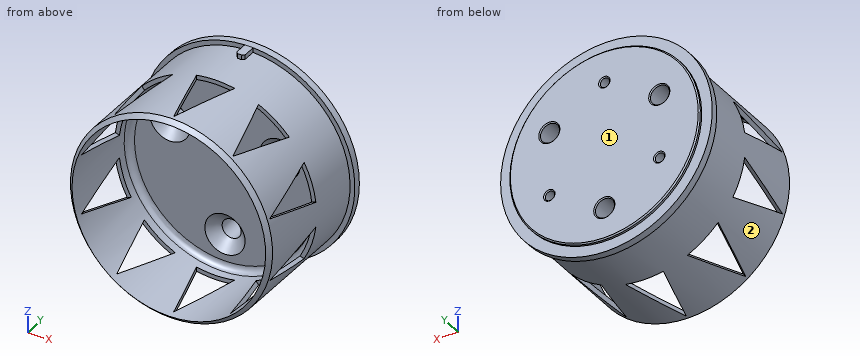
from build123d import *

# Parameters (mm, degrees)
CUT_EXTRUDE_651_DEPTH      = 70.85
PATTERN_CIRCULAR_705_COUNT = 5
SKETCH_7_R                 = 50
EXTRUDE_1_DEPTH            = 5
CUT_EXTRUDE_START          = -1.6
SKETCH_8_R                 = 50
SKETCH_8_R_2               = 45
CUT_EXTRUDE_1_DEPTH        = 1.6
SKETCH_10_R                = 4.5
CUT_EXTRUDE_4_DEPTH        = 97.046863561
SKETCH_10_4_R              = 2.2
CUT_EXTRUDE_5_DEPTH        = 8
CHAMFER_1_SIZE             = 0.5
EXTRUDE_START              = 7
EXTRUDE_2_DEPTH            = 7
CHAMFER_4_SIZE             = 1
CHAMFER_5_SIZE             = 2
CHAMFER_6_SIZE             = 5
CHAMFER_7_SIZE             = 0.6


with BuildPart() as part:
    # Эскиз2 → Revolve 379 (revolve)
    with BuildSketch(Plane.XY, mode=Mode.PRIVATE) as revolve_379_sk:
        with BuildLine():
            Line((0, 0), (-47.75, 0))
            Line((-47.75, 0), (-47.75, -60))
            Line((-47.75, -60), (-45.75, -60))
            Line((-45.75, -60), (-45.75, -21))
            ThreePointArc((-45.75, -21), (-44.871320344, -18.878679656), (-42.75, -18))
            Line((-42.75, -18), (0, -18))
            Line((0, -18), (0, 0))
        make_face()
    revolve(revolve_379_sk.sketch.rotate(Axis((0, 0, 0), (0, 1, 0)), 270), axis=Axis((0, 0, 0), (0, 1, 0)))

    # Эскиз4 → Cut-Extrude 651 (cut, symmetric)
    with BuildSketch(Plane.XY):
        Polygon((-9, -25), (9, -25), (0, -56.5), align=None)
    cut_extrude_651 = extrude(amount=CUT_EXTRUDE_651_DEPTH, both=True, mode=Mode.SUBTRACT)

    # Pattern Circular 705: Cut-Extrude 651 ×5 about axis
    pattern_circular_705_axis = Axis((0, 0, 0), (0, 1, 0))
    for i in range(1, PATTERN_CIRCULAR_705_COUNT):
        add(cut_extrude_651.rotate(pattern_circular_705_axis, i * 360 / PATTERN_CIRCULAR_705_COUNT), mode=Mode.SUBTRACT)

    # Эскиз7 → Бобышка-Вытянуть1 (add)
    with BuildSketch(Plane(origin=(0, 0, 0), x_dir=(1, 0, 0), z_dir=(0, 1, 0))):
        with Locations(Location((0, 0, 0), (0, 0, 270))):
            Circle(SKETCH_7_R)
    extrude(amount=EXTRUDE_1_DEPTH)

    # Эскиз8 → Вырез-Вытянуть1 (cut)
    with BuildSketch(Plane(origin=(0, 5, 0), x_dir=(1, 0, 0), z_dir=(0, 1, 0)).offset(CUT_EXTRUDE_START)):
        with Locations(Location((0, 0, 0), (0, 0, 270))):
            Circle(SKETCH_8_R)
        with Locations(Location((0, 0, 0), (0, 0, 270))):
            Circle(SKETCH_8_R_2, mode=Mode.SUBTRACT)
    extrude(amount=CUT_EXTRUDE_1_DEPTH, mode=Mode.SUBTRACT)

    # Эскиз10 → Вырез-Вытянуть4 (cut, through all)
    with BuildSketch(Plane(origin=(0, 5, 0), x_dir=(1, 0, 0), z_dir=(0, 1, 0))):
        with Locations(Location((0, 30, 0), (0, 0, 270))):
            Circle(SKETCH_10_R)
        with Locations(Location((25.980762114, -15, 0), (0, 0, 270))):
            Circle(SKETCH_10_R)
        with Locations(Location((-25.980762114, -15, 0), (0, 0, 270))):
            Circle(SKETCH_10_R)
    extrude(amount=-CUT_EXTRUDE_4_DEPTH, mode=Mode.SUBTRACT)

    # Эскиз10<4> → Вырез-Вытянуть5 (cut)
    with BuildSketch(Plane(origin=(0, 5, 0), x_dir=(1, 0, 0), z_dir=(0, 1, 0))):
        with Locations(Location((0, -30, 0), (0, 0, 270))):
            Circle(SKETCH_10_4_R)
        with Locations(Location((-25.980762114, 15, 0), (0, 0, 270))):
            Circle(SKETCH_10_4_R)
        with Locations(Location((25.980762114, 15, 0), (0, 0, 270))):
            Circle(SKETCH_10_4_R)
    extrude(amount=-CUT_EXTRUDE_5_DEPTH, mode=Mode.SUBTRACT)

    # Фаска1
    chamfer_1_edges = [part.edges().sort_by_distance(p)[0] for p in [
        (0, 5, -34.5),
        (-25.980762114, 5, 10.5),
        (25.980762114, 5, 10.5),
        (-25.980762114, 5, -17.2),
        (25.980762114, 5, -17.2),
        (0, 5, 27.8),
    ]]
    chamfer(chamfer_1_edges, length=CHAMFER_1_SIZE)

    # Эскиз13 → Бобышка-Вытянуть2 (add)
    with BuildSketch(Plane.XZ.offset(EXTRUDE_START)):
        with BuildLine():
            ThreePointArc((-1.91, 47.711784708), (0, 47.75), (1.91, 47.711784708))
            Line((1.91, 47.711784708), (2, 49.959983987))
            ThreePointArc((2, 49.959983987), (0, 50), (-2, 49.959983987))
            Line((-2, 49.959983987), (-1.91, 47.711784708))
        make_face()
    extrude(amount=-EXTRUDE_2_DEPTH)

    # Фаска4
    chamfer_4_edges = [part.edges().sort_by_distance(p)[0] for p in [
        (-1.955, -7, 48.835884347),
        (1.955, -7, 48.835884347),
    ]]
    chamfer(chamfer_4_edges, length=CHAMFER_4_SIZE)

    # Фаска5
    chamfer_5_edges = [part.edges().sort_by_distance(p)[0] for p in [
        (0, -60, 47.75),
    ]]
    chamfer(chamfer_5_edges, length=CHAMFER_5_SIZE - 0.0001)  # a hair under: the kernel refuses the full size

    # Фаска6
    chamfer_6_edges = [part.edges().sort_by_distance(p)[0] for p in [
        (0, -18, -34.5),
        (-25.980762114, -18, 10.5),
        (25.980762114, -18, 10.5),
    ]]
    chamfer(chamfer_6_edges, length=CHAMFER_6_SIZE)

    # Фаска7
    chamfer_7_edges = [part.edges().sort_by_distance(p)[0] for p in [
        (0, 5, -45),
    ]]
    chamfer(chamfer_7_edges, length=CHAMFER_7_SIZE)


solid = part.part
Read the model definition and answer for the solid it produces. Units are mm, in the model's axes. Face numbers are marked on the shaded views. A direction names the side the tool comes from. Give positions to 0.01 mm unless a question says otherwise; leave off trailing zeros. One line per item, written item: value. Start each with the question number.
(1) A tool of negligible diameter and unlimited length cuts with its end or side. For the marked faces 1 and 2, from which of +Z, -Z, +X, -X, +Y, -Y can it reach the whole face along a straight path? Write none if from no direction.
(2) Find section B-B (y = -36). Give the number of separate pieces and of enclosed holes in the cut face, plus the area to 3 significant figures.
(3) Flat-ended cylindrical pins translate along their axes: pin 1 Ø12 at (y, z) = (-6.5, 29.5) entering from +X; pin 2 Ø3 at (x, y) = (-21.5, -49) entering from +Z; pin 3 Ø1.4 at (x, z) = (4.5, -46.5) entering from -Y. Find the tip coordinate at first contact, or state that the pin passes through.
(4) Find the intervals of material crossed by line 1 (Y direction, x = 39, z = 14); line 2 (Z direction, x = 40, y = -30); line 3 (X direction, y = -3.25, z = 15), in increasing order.
Results below:
1. face 1: +Z, -Z, +X, -X, +Y
1. face 2: -Y
2. separate pieces: 10
2. enclosed holes: 0
2. area: 353 mm^2
3. pin 1: stops at x = 41.57
3. pin 2: stops at z = 43.36
3. pin 3: stops at y = -59.73
4. line 1: y = -18 to 5
4. line 2: z = -26.08 to -22.21, 22.21 to 26.08
4. line 3: x = -45.33 to -30.48, -21.48 to 21.48, 30.48 to 45.33
